```python
from build123d import *

# Parameters (mm, degrees)
F1_DEPTH = 2
F2_R     = 1.5
F3_DEPTH = 25
F4_SIZE  = 0.25


with BuildPart() as f1:
    # F0 (on Right) → F1 (new body)
    with BuildSketch(Plane.YZ):
        Polygon((-1.587713, -2.75), (1.587713, -2.75), (3.175426, 0), (1.587713, 2.75), (-1.587713, 2.75), (-3.175426, 0), align=None)
    extrude(amount=F1_DEPTH)

    # F2 (on Right) → F3 (join)
    with BuildSketch(Plane.YZ):
        Circle(F2_R)
    extrude(amount=-F3_DEPTH)

    # F4
    f4_edges = [f1.edges().sort_by_distance(p)[0] for p in [
        (-25, -1.5, 0),
    ]]
    chamfer(f4_edges, length=F4_SIZE)


solid = f1.part
```
Read the model definition and answer for the solid it produces. Units are mm, in the model's axes. A direction names the side the tool comes from. Coordinates: 2 decimals unless noted, no trailing zeros. Write each loop counter-clockwise with the first axis right and the second up, starting at its lowest first coordinate (ties: lowest second). Pieces come first, ordered by that corner, then holes. Notation, with made-up numbers: (-39.75, 9.5) - (-0.75, 9.5) arc R21 ccw to (-0.75, 42.5) - close; hole circle Ø8 at (-35.75, 3). An arc over 180 degrees is marked (long way). Answer as a JSON object with one key per item and string values. Group by question number.
1. A cutting plane is placed at B-B (x = -11.5). Determine the outline of the cut face in (y, z), plus the area to 3 significant figures.
2. Consider L1, parallel to X at y = 1.75, z = 0.55; L2, parallel to Z at x = -6, y = 1; L3, parallel to Y at x = -19.5, z = 0.3. Determine where each line is inside the solid, lowest interval first. Write a range as [from, to].
3. A cutting plane is placed at A-A (y = 0). Determine the outline of the cut face in (x, z), plus the area to 3 significant figures.
4. Which of the six approach directions +Z, -Z, +X, -X, +Y, -Y give full straight-line access (tool end or side, diameter ignored) to faces 1 (the flat face through (0.99, -2.39, -1.36)), 2 (the flat face through (0, 1.4, 1.3))?
5. Each of these flat-tipped pins is pushed along its axis until it touches: P1, Ø1.5, axis at x = -4.5, z = -1.5, coming from the -Y side; P2, Ø3, axis at x = -13, z = -1.5, coming from the -Y side. Where does it stop, or does it pass through?
6. A cutting plane is placed at C-C (y = -2). Determine the outline of the cut face in (x, z), plus the area to 3 significant figures.
Worked out:
{
 "1": {"outline": "circle Ø3 at (0, 0)", "area": "7.07 mm²"},
 "2": {"L1": "x = [0, 2]", "L2": "z = [-1.12, 1.12]", "L3": "y = [-1.47, 1.47]"},
 "3": {"outline": "(-25, -1.25) - (-24.75, -1.5) - (0, -1.5) - (0, -2.75) - (2, -2.75) - (2, 2.75) - (0, 2.75) - (0, 1.5) - (-24.75, 1.5) - (-25, 1.25) - close", "area": "85.9 mm²"},
 "4": {"face 1": "-Z, +X, -X, -Y", "face 2": "-X"},
 "5": {"P1": "stops at y = -1.3", "P2": "stops at y = -1.5"},
 "6": {"outline": "(0, -2.04) - (2, -2.04) - (2, 2.04) - (0, 2.04) - close", "area": "8.14 mm²"}
}
